```python
from build123d import *

# Parameters (mm, degrees)
F0_R     = 31.75
F1_DEPTH = 44.45
F2_R     = 14.605
F3_DEPTH = 12.7
F4_R     = 5.08


with BuildPart() as f1:
    # F0 (on Top) → F1 (new body)
    with BuildSketch(Plane.XY):
        with Locations((-17.237177, 10.784758)):
            Circle(F0_R)
    extrude(amount=F1_DEPTH)

    # F2 (on face) → F3 (cut)
    with BuildSketch(Plane.XY.offset(44.45)):
        with Locations((-17.237177, 10.784758)):
            Circle(F2_R)
    extrude(amount=-F3_DEPTH, mode=Mode.SUBTRACT)

    # F4
    f4_edges = [f1.edges().sort_by_distance(p)[0] for p in [
        (-48.987177, 10.784758, 44.45),
        (-48.987177, 10.784758, 0),
        (-31.842177, 10.784758, 44.45),
    ]]
    fillet(f4_edges, radius=F4_R)


solid = f1.part
```
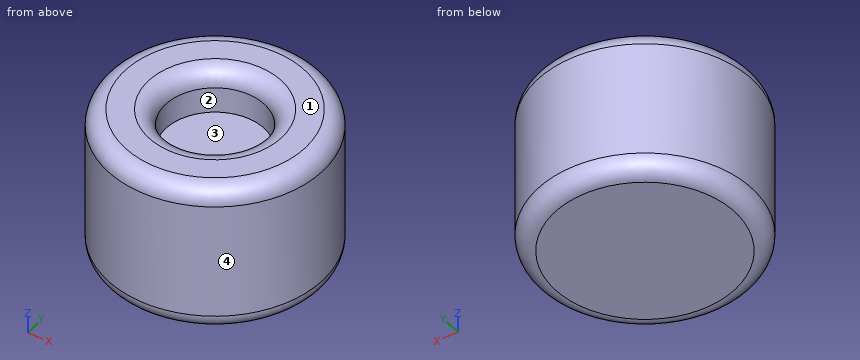
Design review of the part built by this model. Coordinates are the model's own, in mm. Face numbers are marked on the shaded views. Round coordinates to 2 decimals unless told otherwise and drop trailing zeros. Order: outer loops, then holes, each group sorted by start corner. A loop starts at its lowest first (then second) coordinate and runs counter-clockwise, first axis right, second up. Notation, with made-up numbers: (-35.5, 46.25) - (5.5, 46.25) arc R19 ccw to (5.5, 83.25) - close; hole circle Ø1 at (34, 37). An arc over 180 degrees is marked (long way). Return JSON: item names as keys, results as strings.
Q1. For pin 1 Ø2 at (y, z) = (35.5, 27) entering from +X; pin 2 Ø1 at (y, z) = (23, 15.5) entering from -X; pin 3 Ø2 at (x, z) = (6, 24.5) entering from +Y, all flat-tipped, find the tip position at first contact; note any pin that passes through.
Computed values:
{"pin 1": "stops at x = 3.87", "pin 2": "stops at x = -46.75", "pin 3": "stops at y = 33.45"}
Q2. Consider section A-A on z = 34. Write out the cut boundary in (x, y) (3 decimals).
Computed values:
{"outline": "circle Ø63.5 at (-17.237, 10.785); hole circle Ø29.21 at (-17.237, 10.785)"}
Q3. Wall thickness on L1, parallel to Z at x = -25.5, y = 15; L2, parallel to Y at x = -11.5, z = 32; L3, parallel to X at y = 22.5, z = 34: over which ranges is each line inside the solid? List them lowest first. Write a range as [from, to].
Computed values:
{"L1": "z = [0, 31.75]", "L2": "y = [-20.44, -2.65], [24.22, 42.01]", "L3": "x = [-46.75, -25.96], [-8.52, 12.27]"}
Q4. The part is to be moulded in two halves that separate along Y. For the marked faces 1, 2, 3 and 4, say which applies: pulls with the +Y half, pulls with the -Y half, needs draft (parallel to the pull), parting line crosses it, or undercut.
Computed values:
{"face 1": "needs draft", "face 2": "undercut", "face 3": "undercut", "face 4": "parting line crosses it"}
